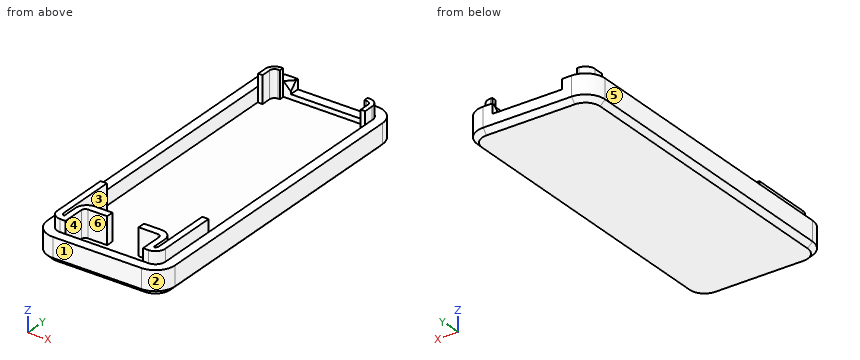
```python
from build123d import *

# Parameters (mm, degrees)
BOSS_EXTRUDE1_DEPTH = 2
BOSS_EXTRUDE2_DEPTH = 5.5
BOSS_EXTRUDE3_DEPTH = 3
SKETCH5_W           = 14.2
SKETCH5_H           = 2
CUT_EXTRUDE1_DEPTH  = 3
CHAMFER1_SIZE       = 1
CHAMFER2_START      = 154
CHAMFER2_DEPTH      = 1.803469575
CHAMFER3_START      = -11.465845015
CHAMFER3_DEPTH      = 10.161362536


with BuildPart() as part:
    # Sketch1 → Boss-Extrude1 (new body)
    with BuildSketch(Plane.XY):
        with BuildLine():
            Line((116.000053406, 143.259475708), (134.000045776, 143.259475708))
            ThreePointArc((134.000045776, 143.259475708), (136.828472901, 142.087902833), (138.000045776, 139.259475708))
            Line((138.000045776, 139.259475708), (138.000045776, 80.259468079))
            ThreePointArc((138.000045776, 80.259468079), (136.828472901, 77.431040954), (134.000045776, 76.259468079))
            Line((134.000045776, 76.259468079), (116.000053406, 76.259468079))
            ThreePointArc((116.000053406, 76.259468079), (113.171626281, 77.431040954), (112.000053406, 80.259468079))
            Line((112.000053406, 80.259468079), (112.000053406, 139.259475708))
            ThreePointArc((112.000053406, 139.259475708), (113.171626281, 142.087902833), (116.000053406, 143.259475708))
        make_face()
    extrude(amount=BOSS_EXTRUDE1_DEPTH)

    # Sketch2 → Boss-Extrude2 (add)
    with BuildSketch(Plane.XY.offset(2)):
        with BuildLine():
            Line((133.600045776, 140.259475708), (134.000045776, 140.259475708))
            ThreePointArc((134.000045776, 140.259475708), (134.707152558, 139.966582489), (135.000045776, 139.259475708))
            Line((135.000045776, 139.259475708), (135.000045776, 137.259475708))
            Line((135.000045776, 137.259475708), (135.900054932, 137.259475708))
            Line((135.900054932, 137.259475708), (135.900054932, 139.259475708))
            ThreePointArc((135.900054932, 139.259475708), (135.343555134, 140.602985066), (134.000045776, 141.159484863))
            Line((134.000045776, 141.159484863), (133.600045776, 141.159484863))
            Line((133.600045776, 141.159484863), (133.600045776, 140.259475708))
        make_face()
        with BuildLine():
            Line((114.10005188, 137.259475708), (115.000053406, 137.259475708))
            Line((115.000053406, 137.259475708), (115.000053406, 139.259475708))
            ThreePointArc((115.000053406, 139.259475708), (115.292946625, 139.966582489), (116.000053406, 140.259475708))
            Line((116.000053406, 140.259475708), (116.400053406, 140.259475708))
            Line((116.400053406, 140.259475708), (116.400053406, 141.159469604))
            Line((116.400053406, 141.159469604), (116.000053406, 141.159469604))
            ThreePointArc((116.000053406, 141.159469604), (114.656549443, 140.602972042), (114.10005188, 139.259468079))
            Line((114.10005188, 139.259468079), (114.10005188, 137.259475708))
        make_face()
        with BuildLine():
            Line((115.300053406, 92.559468079), (114.000048828, 92.559468079))
            Line((114.000048828, 92.559468079), (114.000048828, 80.259475708))
            ThreePointArc((114.000048828, 80.259475708), (114.585836607, 78.845258909), (116.000053406, 78.25947113))
            Line((116.000053406, 78.25947113), (117.100048828, 78.25947113))
            Line((117.100048828, 78.25947113), (117.100048828, 82.759475708))
            ThreePointArc((117.100048828, 82.759475708), (117.334362956, 83.325160054), (117.900047302, 83.559474182))
            Line((117.900047302, 83.559474182), (121.800053406, 83.559474182))
            Line((121.800053406, 83.559474182), (121.800053406, 85.059468079))
            Line((121.800053406, 85.059468079), (118.200050354, 85.059468079))
            ThreePointArc((118.200050354, 85.059468079), (116.573704757, 84.385813675), (115.900050354, 82.759468079))
            Line((115.900050354, 82.759468079), (115.900050354, 79.566648196))
            ThreePointArc((115.900050354, 79.566648196), (115.470902134, 79.801211675), (115.300053406, 80.259468079))
            Line((115.300053406, 80.259468079), (115.300053406, 92.559468079))
        make_face()
        with BuildLine():
            Line((128.200045776, 85.059468079), (128.200045776, 83.559458923))
            Line((128.200045776, 83.559458923), (132.10005188, 83.559458923))
            ThreePointArc((132.10005188, 83.559458923), (132.665730831, 83.32514703), (132.900042725, 82.759468079))
            Line((132.900042725, 82.759468079), (132.900042725, 78.25947113))
            Line((132.900042725, 78.25947113), (134.000045776, 78.25947113))
            ThreePointArc((134.000045776, 78.25947113), (135.414257181, 78.845256674), (136.000042725, 80.259468079))
            Line((136.000042725, 80.259468079), (136.000042725, 92.559468079))
            Line((136.000042725, 92.559468079), (134.700045776, 92.559468079))
            Line((134.700045776, 92.559468079), (134.700045776, 80.259468079))
            ThreePointArc((134.700045776, 80.259468079), (134.529197048, 79.801211675), (134.100048828, 79.566648196))
            Line((134.100048828, 79.566648196), (134.100048828, 82.759468079))
            ThreePointArc((134.100048828, 82.759468079), (133.426394425, 84.385813675), (131.800048828, 85.059468079))
            Line((131.800048828, 85.059468079), (128.200045776, 85.059468079))
        make_face()
    extrude(amount=BOSS_EXTRUDE2_DEPTH)


with BuildPart() as boss_extrude3_tool:
    # Sketch3 → Boss-Extrude3 (new body)
    with BuildSketch(Plane.XY.offset(2)):
        with BuildLine():
            Line((116.000053406, 76.259468079), (134.000045776, 76.259468079))
            ThreePointArc((134.000045776, 76.259468079), (136.828472901, 77.431040954), (138.000045776, 80.259468079))
            Line((138.000045776, 80.259468079), (138.000045776, 139.259475708))
            ThreePointArc((138.000045776, 139.259475708), (136.828472901, 142.087902833), (134.000045776, 143.259475708))
            Line((134.000045776, 143.259475708), (116.000053406, 143.259475708))
            ThreePointArc((116.000053406, 143.259475708), (113.171626281, 142.087902833), (112.000053406, 139.259475708))
            Line((112.000053406, 139.259475708), (112.000053406, 80.259468079))
            ThreePointArc((112.000053406, 80.259468079), (113.171626281, 77.431040954), (116.000053406, 76.259468079))
        make_face()
        with BuildLine():
            Line((116.000053406, 78.259468079), (134.000045776, 78.259468079))
            ThreePointArc((134.000045776, 78.259468079), (135.414259339, 78.845254516), (136.000045776, 80.259468079))
            Line((136.000045776, 80.259468079), (136.000045776, 139.259475708))
            ThreePointArc((136.000045776, 139.259475708), (135.414259339, 140.67368927), (134.000045776, 141.259475708))
            Line((134.000045776, 141.259475708), (116.000053406, 141.259475708))
            ThreePointArc((116.000053406, 141.259475708), (114.585839843, 140.67368927), (114.000053406, 139.259475708))
            Line((114.000053406, 139.259475708), (114.000053406, 80.259468079))
            ThreePointArc((114.000053406, 80.259468079), (114.585839843, 78.845254516), (116.000053406, 78.259468079))
        make_face(mode=Mode.SUBTRACT)
    extrude(amount=BOSS_EXTRUDE3_DEPTH)


with BuildPart() as part_1:
    add(part.part)


with BuildPart() as part_2:
    # Boss-Extrude3: joined with boss_extrude3_tool
    add(part_1.part.fuse(boss_extrude3_tool.part, tol=0.00001))

    # Sketch5 → Cut-Extrude1 (cut)
    with BuildSketch(Plane(origin=(0, 143.259475708, 0), x_dir=(1, 0, 0), z_dir=(0, 1, 0))):
        with Locations((125.000049591, -4)):
            Rectangle(SKETCH5_W, SKETCH5_H)
    extrude(amount=-CUT_EXTRUDE1_DEPTH, mode=Mode.SUBTRACT)

    # Chamfer1
    chamfer1_edges = [part_2.edges().sort_by_distance(p)[0] for p in [
        (138.000045776, 109.759471893, 0),
        (136.828472901, 77.431040954, 0),
        (125.000049591, 76.259468079, 0),
        (113.171626281, 77.431040954, 0),
        (112.000053406, 109.759471893, 0),
        (113.171626281, 142.087902833, 0),
        (125.000049591, 143.259475708, 0),
        (136.828472901, 142.087902833, 0),
    ]]
    chamfer(chamfer1_edges, length=CHAMFER1_SIZE)

    # Chamfer2: read off the stored shape, not the designer's step
    # Chamfer2 outline → Chamfer2 (cut)
    with BuildSketch(Plane(origin=(0, 0, 0), x_dir=(0.8164965809277274, -0.4082482904638596, 0.4082482904638638), z_dir=(0.5773502691896238, 0.5773502691896238, -0.5773502691896297)).offset(CHAMFER2_START)):
        Polygon((51.619168378, -104.481727258), (53.456285686, -103.421067086), (51.619168378, -102.360406914), align=None)
    extrude(amount=CHAMFER2_DEPTH, mode=Mode.SUBTRACT)

    # Chamfer3: read off the stored shape, not the designer's step
    # Chamfer3 outline → Chamfer3 (cut)
    with BuildSketch(Plane(origin=(0, 0, 0), x_dir=(0.8164965809277249, 0.4082482904638619, -0.4082482904638661), z_dir=(0.5773502691896272, -0.5773502691896221, 0.5773502691896281)).offset(CHAMFER3_START)):
        Polygon((152.505057835, 104.481727258), (150.667940528, 103.421067086), (152.505057835, 102.360406914), align=None)
    extrude(amount=CHAMFER3_DEPTH, mode=Mode.SUBTRACT)


solid = part_2.part
```
Here's how the part is built. I have some questions about the finished solid (model axes, mm). Face numbers are marked on the shaded views. A direction names the side the tool comes from. Coordinates: 2 decimals unless noted, no trailing zeros. Write each loop counter-clockwise with the first axis right and the second up, starting at its lowest first coordinate (ties: lowest second). Pieces come first, ordered by that corner, then holes. Notation, with made-up numbers: (59.25, -25) -> (73.25, -25) arc R19 ccw to (73.25, -3) -> close; hole circle Ø2 at (-19, 40). An arc over 180 degrees is marked (long way). Use a Markdown table: item, result. Add a question column.
(1) We'd pull the mould along X, two halves only. Please class the marked faces 1, 2, 3 and 4: +X half, -X half, draft (parallel to the pull), parting line (faces both ways), or undercut.
(2) For the marked faces 5 and 6, which set-ups out of +Z, -Z, +X, -X, +Y, -Y let a thin tool reach every point of the face, with its end or its side?
(3) If we section it at B-B, the plane z = 6: State how many separate pieces and enclosed holes the cut face has, and give its area (3 significant figures).
(4) If we section it at D-D, the plane y = 88.5: Write out the boundary of the cut face in (x, z), and give its area (3 significant figures).
(5) If we section it at A-A, the plane y = 125: Write out the boundary of the cut face in (x, z), and give its area (3 significant figures).
(6) I'm going to push flat-ended pins straight in: P1, Ø1.5, axis at x = 120, y = 122.5, coming from the +Z side; P2, Ø1, axis at y = 142, z = 4.5, coming from the +X side; P3, Ø1, axis at x = 122, y = 142.5, coming from the +Z side. Where does each tip first touch, or does it pass through?
(7) If we section it at C-C, the plane x = 127.5: Write out the boundary of the cut face in (y, z).
(8) Please list where these lines run through material, in increasing order: line 1 (Y direction, x = 132, z = 4.25); line 2 (Y direction, x = 119.5, z = 2.5); line 3 (X direction, y = 89, z = 4.75).
Outcome:
| question | item | result |
|---|---|---|
| 1 | face 1 | draft |
| 1 | face 2 | +X half |
| 1 | face 3 | undercut |
| 1 | face 4 | undercut |
| 2 | face 5 | +Z, -Z, -X, +Y, -Y |
| 2 | face 6 | +Z |
| 3 | separate pieces | 4 |
| 3 | enclosed holes | 0 |
| 3 | area | 74.1 mm^2 |
| 4 | outline | (112, 1) -> (113, 0) -> (137, 0) -> (138, 1) -> (138, 5) -> (136, 5) -> (136, 7.5) -> (134.7, 7.5) -> (134.7, 2) -> (115.3, 2) -> (115.3, 7.5) -> (114, 7.5) -> (114, 5) -> (112, 5) -> close |
| 4 | area | 77.3 mm^2 |
| 5 | outline | (112, 1) -> (113, 0) -> (137, 0) -> (138, 1) -> (138, 5) -> (136, 5) -> (136, 2) -> (114, 2) -> (114, 5) -> (112, 5) -> close |
| 5 | area | 63.0 mm^2 |
| 6 | P1 | stops at z = 2 |
| 6 | P2 | stops at x = 137.31 |
| 6 | P3 | stops at z = 3 |
| 7 | outline | (76.26, 1) -> (77.26, 0) -> (142.26, 0) -> (143.26, 1) -> (143.26, 3) -> (141.26, 3) -> (141.26, 2) -> (78.26, 2) -> (78.26, 5) -> (76.26, 5) -> close |
| 8 | line 1 | y = 76.26 to 78.26, 83.56 to 85.05 |
| 8 | line 2 | y = 76.26 to 78.26, 83.56 to 85.06, 141.26 to 143.26 |
| 8 | line 3 | x = 112 to 115.3, 134.7 to 138 |
